Autodesk Inventor part; units mm, degrees
ref_plane "YZ Plane" through (0, 0, 0) normal (1, 0, 0) x (0, 1, 0)
ref_plane "XZ Plane" through (0, 0, 0) normal (0, 1, 0) x (-1, 0, 0)
ref_plane "XY Plane" through (0, 0, 0) normal (0, 0, 1) x (1, 0, 0)
sketch "Sketch1" plane through (0, 0, 0) normal (0, 1, 0) x (-1, 0, 0)
  line L0 (0, 0) -> (30, 0)
  line L1 (30, 0) -> (30, -20)
  line L2 (30, -20) -> (0, -20)
  line L3 (0, -20) -> (0, 0)
  line L4 (30, -10) -> (0, -10)
  line L5 (15, 0) -> (15, -20)
  circle A0 centre (25, -10) radius 2
  circle A1 centre (15, -38) radius 2.5
  line L6 (30, -20) -> (19.5, -41)
  circle A2 centre (5, -10) radius 2
  line L7 (0, -20) -> (10.5, -41)
  arc A3 (10.5, -41) -> (19.5, -41) centre (15, -38.75) ccw
  line L8 (30, 0) -> (0, 0)
  circle A4 centre (15, 18) radius 2.5
  line L9 (30, 0) -> (19.5, 21)
  line L10 (0, 0) -> (10.5, 21)
  arc A5 (19.5, 21) -> (10.5, 21) centre (15, 18.75) ccw
  dimension "d0" = 20
  dimension "d1" = 30
  dimension "d2" = 5
  dimension "d3" = 4
  dimension "d5" = 18
  dimension "d6" = 5
  dimension "d7" = 21
  dimension "d8" = 10.5
extrude "Extrusion1" add sketch "Sketch1" along normal blind 1 contours L10 A5 L9 L0 | L0 L5 L4 A2 L3 | L0 L1 L4 A0 L5 | L4 A2 L5 L2 L3 | L4 A0 L1 L2 L5 | L2 L6 A3 L7
properties part number "Platte2"
Part model, mm, in its own coordinate system. Give positions to 0.01 mm unless a question says otherwise; leave off trailing zeros. Loops run counter-clockwise (first coordinate to the right, second up) from the corner with the lowest first, then second, coordinate; pieces in that order, holes last. Notation, with made-up numbers: M 34.25,60 L 84.25,60 A22 cw 84.25,81 Z; hole C 80,57.25 d3. An arc over 180 degrees is marked long. Put each result on its own line as item: value. Start each with the question number.
1) Probe probe 1 along X at (y, z) = (0.4, -10); probe 2 along Z at (x, y) = (-15.25, 0.8); probe 3 along Z at (x, y) = (-24.75, 0.4). List the from-to ranges inside material, lowest first.
2) Saw through at A-A (z = -38). List the corners of the cut face in (x, y), then the cut area to 3 significant figures.
3) Saw through at C-C (y = 0.6). List the corners of the cut face in (x, z).
4) Saw through at D-D (z = -10). List the corners of the cut face in (x, y), then the cut area to 3 significant figures.
5) Saw through at B-B (x = -5). List the corners of the cut face in (y, z), then the cut area to 3 significant figures.
6) Pull direction Z, two halves, no side cores. Call faces 1 (the cylindrical face through (-14.92, 0.49, 23.78)), 2 (the cylindrical face through (-23.526, 0.493, -11.352)), 3 (the flat face through (-24.8, 0.5, -30.4)): +Z half, -Z half, draft (parallel to the pull), parting line (faces both ways), or undercut.
Numbers:
1. probe 1: -30 to -27, -23 to -7, -3 to 0
1. probe 2: -43.77 to -40.49, -35.51 to 15.51, 20.49 to 23.77
1. probe 3: -30.5 to -11.98, -8.02 to 10.5
2. outline: M -21,0 L -17.5,0 L -17.5,1 L -21,1 Z; M -12.5,0 L -9,0 L -9,1 L -12.5,1 Z
2. area: 7.00 mm^2
3. outline: M -30,-20 L -19.5,-41 A5.03 ccw -10.5,-41 L 0,-20 L 0,0 L -10.5,21 A5.03 ccw -19.5,21 L -30,0 Z; hole C -25,-10 d4; hole C -15,-38 d5; hole C -15,18 d5; hole C -5,-10 d4
4. outline: M -30,0 L -27,0 L -27,1 L -30,1 Z; M -23,0 L -7,0 L -7,1 L -23,1 Z; M -3,0 L 0,0 L 0,1 L -3,1 Z
4. area: 22.0 mm^2
5. outline: M 0,-30 L 1,-30 L 1,-12 L 0,-12 Z; M 0,-8 L 1,-8 L 1,10 L 0,10 Z
5. area: 36.0 mm^2
6. face 1: +Z half
6. face 2: undercut
6. face 3: -Z half
